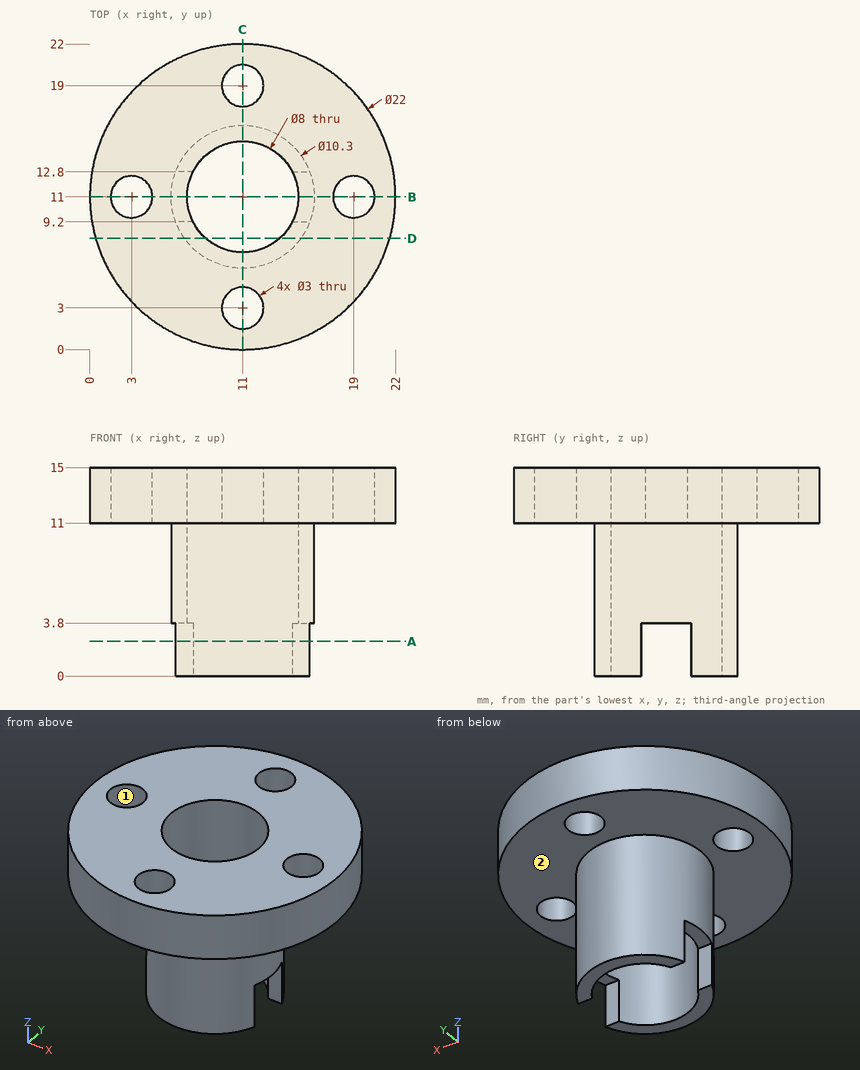
Input: dimensioned drawing with shaded views. Units: mm. Origin: part minimum x, y, z. A direction names the side the tool comes from. Round coordinates to 2 decimals unless told otherwise and drop trailing zeros. Write each loop counter-clockwise with the first axis right and the second up, starting at its lowest first coordinate (ties: lowest second). Pieces come first, ordered by that corner, then holes. Notation, with made-up numbers: (53.25, -26) -> (60.25, -26) arc R32 ccw to (60.25, 0) -> close; hole circle Ø2 at (69.25, -39). An arc over 180 degrees is marked (long way). Use CSV: the item, a comma, the result in double quotes. Start each with the question number.
Q1. Section B-B (y = 11). Return loops of the section in (x, z).
Q2. First-contact query: pin 1 Ø1.8 at (x, y) = (11, 3) entering from +Z; pin 2 Ø4 at (x, z) = (11, 2) entering from +Y; pin 3 Ø4 at (x, y) = (11, 19) entering from +Z; pin 4 Ø1.5 at (y, z) = (7.5, 8) entering from +X. Flat tips, straight axial feed; report the tip coordinate or a pass-through.
Q3. Section D-D (y = 8). Return loops of the section in (x, z).
Q4. Section A-A (z = 2.5). Return loops of the section in (x, y).
Q5. Reachability of the marked faces 1 and 2 from +Z, -Z, +X, -X, +Y, -Y: full face, straight path, thin tool, end or side. Return the list, or none.
Q6. Section C-C (x = 11). Return loops of the section in (y, z).
Q7. Line query: L1, parallel to Y at x = 11, z = 12.9; L2, parallel to Z at x = 20.5, y = 11.75; L3, parallel to Y at x = 11, z = 9.5. Output: solid intervals per line, ascending.
Result sheet:
1,outline,"(0, 11) -> (1.5, 11) -> (1.5, 15) -> (0, 15) -> close; (4.5, 11) -> (5.85, 11) -> (5.85, 3.8) -> (7, 3.8) -> (7, 15) -> (4.5, 15) -> close; (15, 3.8) -> (16.15, 3.8) -> (16.15, 11) -> (17.5, 11) -> (17.5, 15) -> (15, 15) -> close; (20.5, 11) -> (22, 11) -> (22, 15) -> (20.5, 15) -> close"
2,pin 1,"through"
2,pin 2,"y = 16.15"
2,pin 3,"z = 15"
2,pin 4,"x = 15.35"
3,outline,"(0.42, 11) -> (6.81, 11) -> (6.81, 0) -> (8.35, 0) -> (8.35, 15) -> (0.42, 15) -> close; (13.65, 0) -> (15.19, 0) -> (15.19, 11) -> (21.58, 11) -> (21.58, 15) -> (13.65, 15) -> close"
4,outline,"(6.17, 9.2) arc R5.15 ccw to (15.83, 9.2) -> (14.57, 9.2) arc R4 cw to (7.43, 9.2) -> close; (6.17, 12.8) -> (7.43, 12.8) arc R4 cw to (14.57, 12.8) -> (15.83, 12.8) arc R5.15 ccw to start"
5,face 1,"+Z, -Z"
5,face 2,"-Z"
6,outline,"(0, 11) -> (1.5, 11) -> (1.5, 15) -> (0, 15) -> close; (4.5, 11) -> (5.85, 11) -> (5.85, 0) -> (7, 0) -> (7, 15) -> (4.5, 15) -> close; (15, 0) -> (16.15, 0) -> (16.15, 11) -> (17.5, 11) -> (17.5, 15) -> (15, 15) -> close; (20.5, 11) -> (22, 11) -> (22, 15) -> (20.5, 15) -> close"
7,L1,"0 to 1.5, 4.5 to 7, 15 to 17.5, 20.5 to 22"
7,L2,"11 to 15"
7,L3,"5.85 to 7, 15 to 16.15"
